Geometry: see drawing. Coordinates: mm, zero at the bounding-box minimum. Give positions to 0.01 mm unless a question says otherwise; leave off trailing zeros. Order: outer loops, then holes, each group sorted by start corner. A loop starts at its lowest first (then second) coordinate and runs counter-clockwise, first axis right, second up. Notation, with made-up numbers: (76, 54) - (91, 54) arc R20 cw to (91, 89) - close; hole circle Ø2 at (67.5, -7.5). An arc over 180 degrees is marked (long way). One line per question, with ' | ' between items. Start each with the question number.
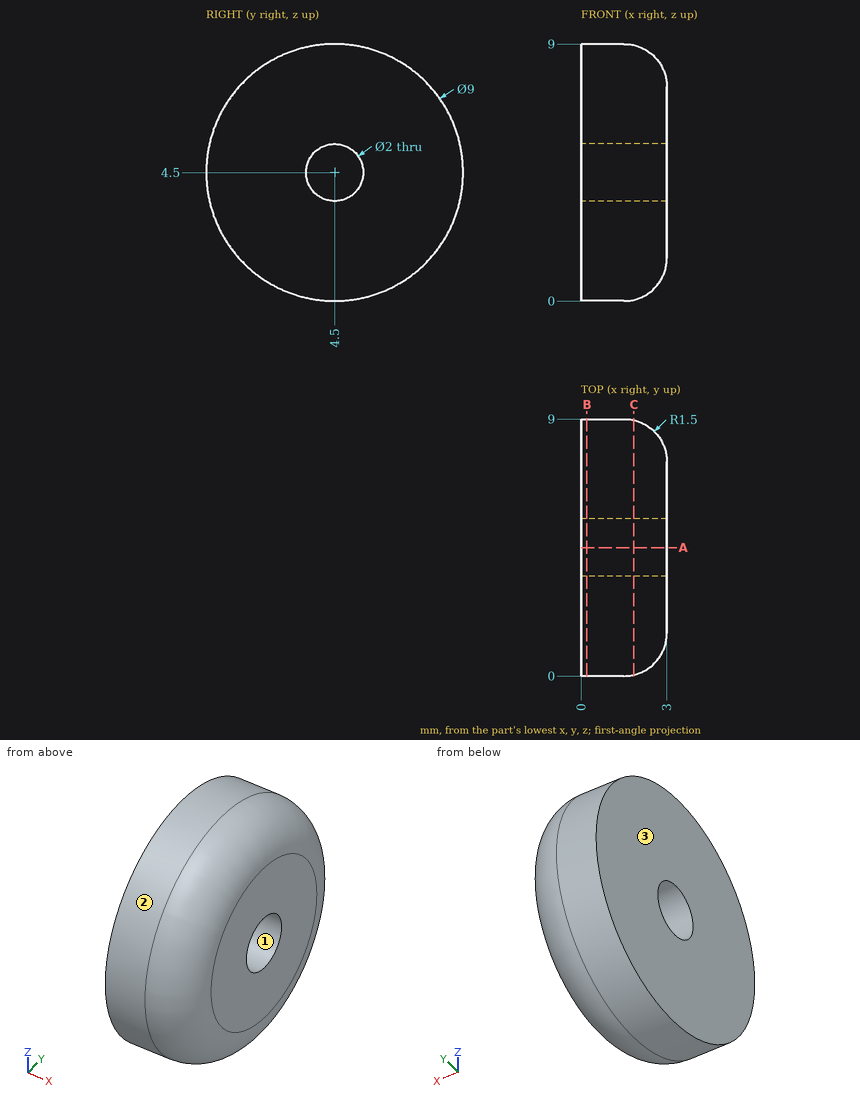
(1) Contact query for flat-ended pins moving along their axis: P1, Ø1.5, axis at x = 1, y = 1.5, coming from the -Z side; P2, Ø1.5, axis at x = 2, y = 1.5, coming from the -Z side; P3, Ø3, axis at y = 4, z = 8, coming from the +X side. Output: stop coordinate, or through.
(2) Cut plane B-B, the plane x = 0.2. Return the cut outline in (y, z).
(3) Cut plane A-A, the plane y = 4.5. Return the cut outline in (x, z), plus the area to 3 significant figures.
(4) Pull-direction query (Y, two-part tool) for the marked faces 1, 2 and 3; classes: +Y half, -Y half, draft (parallel to the pull), parting line (faces both ways), or undercut.
(5) Cut plane C-C, the plane x = 1.85. Return the cut outline in (y, z).
(6) Material intervals for line 1 along Z through (x, y) = (0.6, 4.5); line 2 along Z through (x, y) = (2.25, 4.5); line 3 along Y through (x, z) = (2.3, 6.5), sorted ascending. Write a range as from..to.
Results are:
1) P1: z = 0.6 | P2: z = 0.65 | P3: x = 3
2) outline: circle Ø9 at (4.5, 4.5); hole circle Ø2 at (4.5, 4.5)
3) outline: (0, 0) - (1.5, 0) arc R1.5 ccw to (3, 1.5) - (3, 3.5) - (0, 3.5) - close; (0, 5.5) - (3, 5.5) - (3, 7.5) arc R1.5 ccw to (1.5, 9) - (0, 9) - close | area: 20.0 mm2
4) face 1: undercut | face 2: parting line | face 3: draft
5) outline: circle Ø8.92 at (4.5, 4.5); hole circle Ø2 at (4.5, 4.5)
6) line 1: 0..3.5, 5.5..9 | line 2: 0.2..3.5, 5.5..8.8 | line 3: 0.73..8.27
